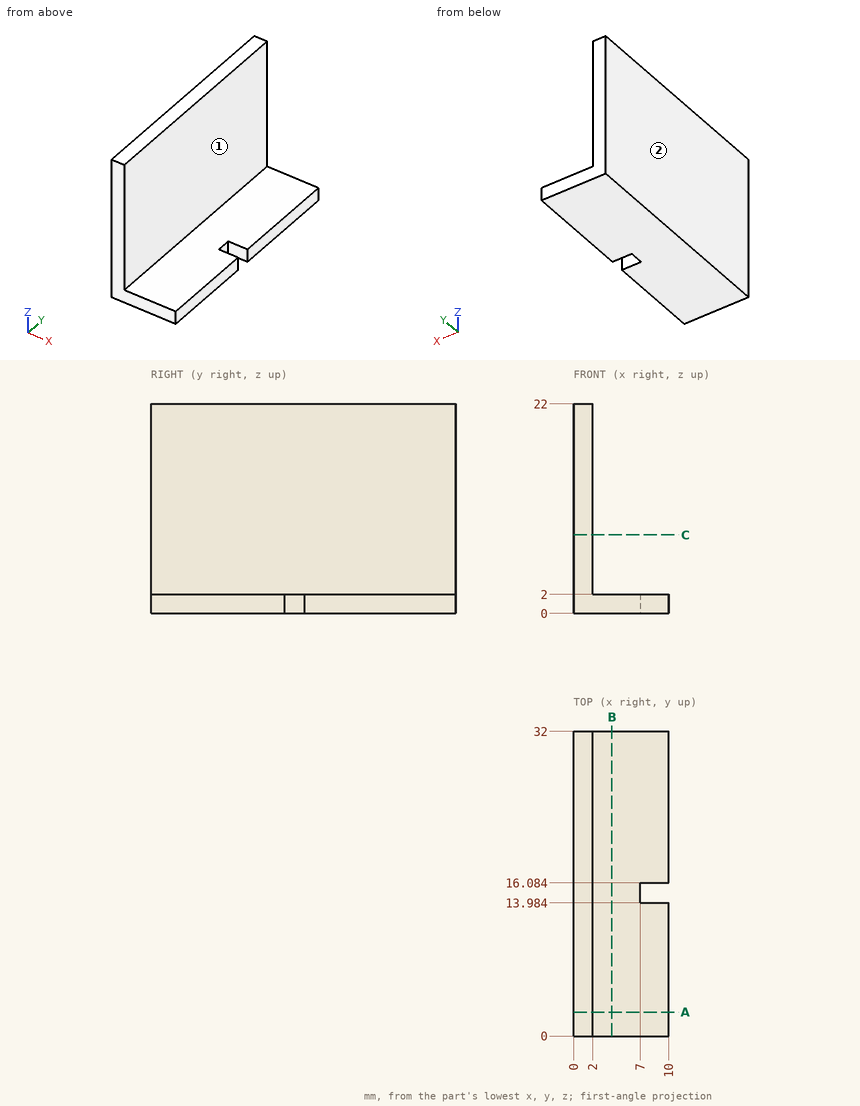
Source: three-view drawing plus pictorial views. Frame: mm from the lowest corner of the part. A direction names the side the tool comes from. Round coordinates to 2 decimals unless told otherwise and drop trailing zeros. Loops run counter-clockwise (first coordinate to the right, second up) from the corner with the lowest first, then second, coordinate; pieces in that order, holes last. Notation, with made-up numbers: (22.25, -13) - (36.25, -13) arc R25 ccw to (36.25, 9) - close; hole circle Ø1 at (89, -39.5). An arc over 180 degrees is marked (long way). Write each question's results on one line, items separated by ' | '. Start each with the question number.
1) Cut plane B-B on x = 4. Return loops of the section in (y, z).
2) Cut plane A-A on y = 2.5. Return loops of the section in (x, z).
3) Cut plane C-C on z = 8.25. Return loops of the section in (x, y).
4) First-contact query: P1, Ø1, axis at x = 8.5, y = 23.5, coming from the +Z side; P2, Ø10, axis at y = 16, z = 13.5, coming from the +X side; P3, Ø1, axis at y = 15.5, z = 1.5, coming from the +X side. Flat tips, straight axial feed; report the tip coordinate or a pass-through.
5) Line query: probe 1 along Z at (x, y) = (2.25, 12). Output: solid intervals per line, ascending. Write a range as [from, to].
6) Access query for the marked faces 1 and 2. Directions: +Z, -Z, +X, -X, +Y, -Y. A direction counts if a zero-diameter tool reaches every point of the face in a straight line with its end or side. Return the directions, or none.
Verdict:
1) outline: (0, 0) - (32, 0) - (32, 2) - (0, 2) - close
2) outline: (0, 0) - (10, 0) - (10, 2) - (2, 2) - (2, 22) - (0, 22) - close
3) outline: (0, 0) - (2, 0) - (2, 32) - (0, 32) - close
4) P1: stops at z = 2 | P2: stops at x = 2 | P3: stops at x = 7
5) probe 1: z = [0, 2]
6) face 1: +Z, +X, +Y, -Y | face 2: +Z, -Z, -X, +Y, -Y
